Geometry: see drawing. Coordinates: mm, zero at the bounding-box minimum. A direction names the side the tool comes from. Round coordinates to 2 decimals unless told otherwise and drop trailing zeros. Order: outer loops, then holes, each group sorted by start corner. A loop starts at its lowest first (then second) coordinate and runs counter-clockwise, first axis right, second up. Notation, with made-up numbers: (30.5, 13.5) -> (68.5, 13.5) arc R11 ccw to (68.5, 32.5) -> close; hole circle Ø6 at (54.5, 9.5). An arc over 180 degrees is marked (long way). Put each result on its own line as item: value.
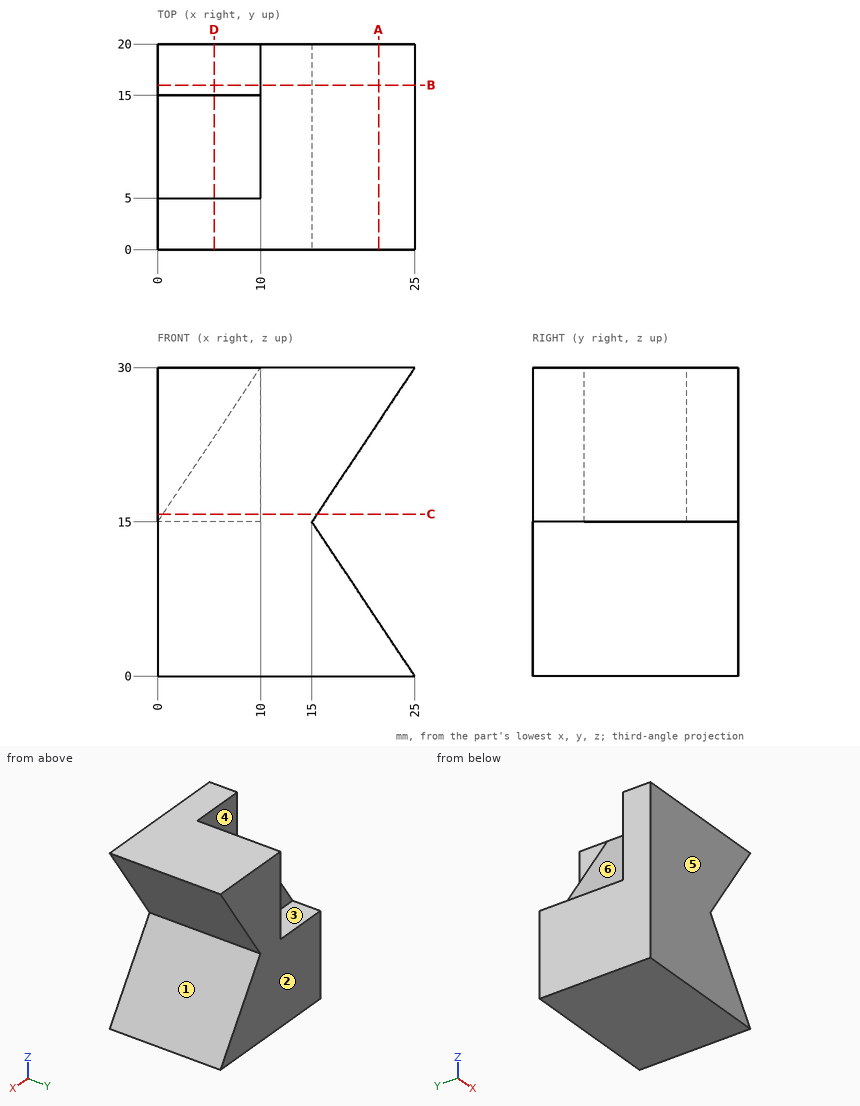
1. Cut plane A-A on x = 21.5. Return loops of the section in (y, z).
Ans:
outline: (0, 0) -> (20, 0) -> (20, 5.25) -> (0, 5.25) -> close; (0, 24.75) -> (20, 24.75) -> (20, 30) -> (0, 30) -> close
2. Cut plane D-D on x = 5.5. Return loops of the section in (y, z).
Ans:
outline: (0, 0) -> (20, 0) -> (20, 15) -> (15, 15) -> (15, 23.25) -> (5, 23.25) -> (5, 30) -> (0, 30) -> close
3. Draft query along Y for the marked faces 4, 5 and 6. Return one class per face: +Y half, -Y half, draft (parallel to the pull), parting line (faces both ways), or undercut.
Ans:
face 4: +Y half
face 5: -Y half
face 6: draft
4. Material intervals for probe 1 along Y at (x, z) = (9, 27.25); probe 2 along Z at (x, y) = (17.5, 2.5), sorted ascending.
Ans:
probe 1: 0 to 15
probe 2: 0 to 11.25, 18.75 to 30
5. Set-up query: the marked faces 1, 2 and 3. Return all of +Z, -Z, +X, -X, +Y, -Y with unobstructed straight access to the full face (end or side cutting, diameter ignored); none if empty.
Ans:
face 1: +X, +Y, -Y
face 2: +Z, -Z, +X, -X, +Y
face 3: +Z, -X, +Y
6. Cut plane C-C on z = 15.75. Return loops of the section in (x, y).
Ans:
outline: (0, 0) -> (15.5, 0) -> (15.5, 20) -> (10, 20) -> (10, 15) -> (0.5, 15) -> (0.5, 5) -> (0, 5) -> close
7. Cut plane B-B on y = 16. Return loops of the section in (x, z).
Ans:
outline: (0, 0) -> (25, 0) -> (15, 15) -> (25, 30) -> (10, 30) -> (10, 15) -> (0, 15) -> close
8. Contact query for flat-ended pins moving along their axis: P1, Ø5, axis at x = 19.5, z = 12.5, coming from the +Y side; P2, Ø4, axis at y = 14.5, z = 20, coming from the +X side; P3, Ø1.5, axis at y = 18, z = 21.5, coming from the -X side; P4, Ø1.5, axis at x = 4.5, y = 17, coming from the +Z side. Output: stop coordinate, or through.
Ans:
P1: y = 20
P2: x = 19.67
P3: x = 10
P4: z = 15
